Here's how the part is built. I have some questions about the finished solid (model axes, mm). A direction names the side the tool comes from. Give positions to 0.01 mm unless a question says otherwise; leave off trailing zeros. Order: outer loops, then holes, each group sorted by start corner. A loop starts at its lowest first (then second) coordinate and runs counter-clockwise, first axis right, second up. Notation, with made-up numbers: M 55.5,11 L 82.5,11 A23 ccw 82.5,34 Z; hole C 20.25,48 d7. An arc over 180 degrees is marked long. Use one line per item in the form item = value.
from build123d import *

# Parameters (mm, degrees)
ESBO_O1_W             = 10
ESBO_O1_H             = 10
EXTRUS_O1_DEPTH       = 40
ESBO_O2_W             = 14.229592149
ESBO_O2_H             = 10.020208066
EXTRUS_O2_DEPTH       = 3
ESBO_O3_R             = 14.5
CORTE_EXTRUS_O1_DEPTH = 23
ESBO_O4_R             = 13
CORTE_EXTRUS_O2_DEPTH = 23


with BuildPart() as part:
    # Esboço1 → Extrusão1 (new body)
    with BuildSketch(Plane(origin=(0, 0, 0), x_dir=(0, 0, -1), z_dir=(1, 0, 0))):
        Rectangle(ESBO_O1_W, ESBO_O1_H)
    extrude(amount=-EXTRUS_O1_DEPTH)

    # Esboço2 → Extrusão2 (add)
    with BuildSketch(Plane(origin=(0, 0, 0), x_dir=(0, 0, -1), z_dir=(1, 0, 0))):
        with Locations((2.114796075, -0.010104033)):
            Rectangle(ESBO_O2_W, ESBO_O2_H)
    extrude(amount=-EXTRUS_O2_DEPTH)

    # Esboço3 → Corte-extrusão1 (cut)
    with BuildSketch(Plane(origin=(0, 0, 0), x_dir=(0, 0, -1), z_dir=(1, 0, 0))):
        with Locations((21.55, 0)):
            Circle(ESBO_O3_R)
    extrude(amount=-CORTE_EXTRUS_O1_DEPTH, mode=Mode.SUBTRACT)

    # Esboço4 → Corte-extrusão2 (cut)
    with BuildSketch(Plane.XY.offset(5)):
        with Locations((-49, 0)):
            Circle(ESBO_O4_R)
    extrude(amount=-CORTE_EXTRUS_O2_DEPTH, mode=Mode.SUBTRACT)


solid = part.part
Q1. Thinking about a two-plate mould opening in Y: for faces 1 (the face through (-36, 0, 0)), 2 (the face through (-1, -5.02, -1)), 3 (the face through (-3, 0, -6)), which applies, +Y half, -Y half, draft (parallel to the pull), parting line (faces both ways), or undercut?
Found:
face_1 = undercut
face_2 = -Y half
face_3 = draft
Q2. On a 3-axis mill with a long thin cutter (end or side, diameter ignored), from which of +Z, -Z, +X, -X, +Y, -Y can I reach the whole of each face in a straight line? I mean faces 4 (the face through (-20, 0, -5)), 5 (the face through (-1.48, 0.06, -7.05)). Say none if no direction works.
Found:
face_4 = -Z, -X, +Y, -Y
face_5 = -Z, +X, -X
Q3. I want a section at C-C on y = 1. Write out the boundary of the cut face in (x, z).
Found:
outline = M -36.04,-5 L -3,-5 L -3,-7.08 L 0,-7.08 L 0,5 L -36.04,5 Z
Q4. I'm going to push flat-ended pins straight in: pin 1 Ø3 at (x, y) = (-10, -3) entering from -Z; pin 2 Ø6 at (y, z) = (3.5, -1.5) entering from -X; pin 3 Ø5 at (x, z) = (-14, 1.5) entering from -Y. Where does each tip first touch, or does it pass through?
Found:
pin_1 = -5
pin_2 = -37
pin_3 = -5
Q5. I want a section at B-B on x = -33.5. Write out the boundary of the cut face in (y, z).
Found:
outline = M -5,-5 L 5,-5 L 5,5 L -5,5 Z
Q6. I need wall thicknesses on L1, parallel to Z at x = -7, y = 1.75; L2, parallel to X at y = 4, z = -4. Which ranges of each line are inside material? Lowest first, please.
Found:
L1 = -5 to 5
L2 = -36.63 to 0
